Verification items for the finished model (mm, model axes). Face numbers are marked on the shaded views. Give positions to 0.01 mm unless a question says otherwise; leave off trailing zeros. Order: outer loops, then holes, each group sorted by start corner. A loop starts at its lowest first (then second) coordinate and runs counter-clockwise, first axis right, second up. Notation, with made-up numbers: M 16.25,59.25 L 70.25,59.25 A18 ccw 70.25,85.25 Z; hole C 3,-32 d3. An arc over 180 degrees is marked long. Answer as a JSON object with one key per item and string values.
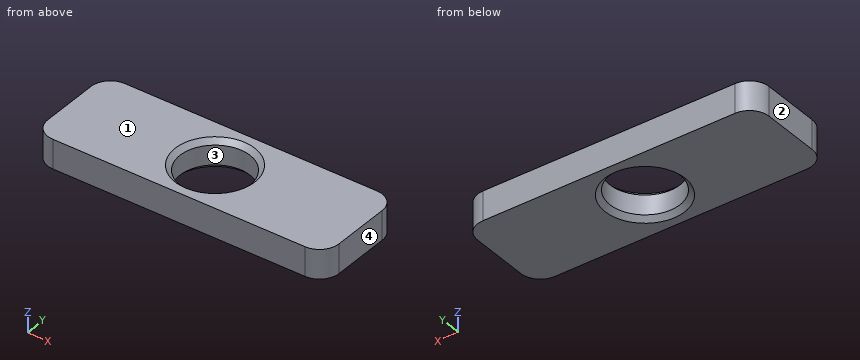
```python
from build123d import *

# Parameters (mm, degrees)
F0_W     = 300
F0_H     = 100
F0_R     = 36.023604
F1_DEPTH = 30
F2_R     = 20
F3_SIZE  = 5


with BuildPart() as f1:
    # F0 (on Top) → F1 (new body)
    with BuildSketch(Plane.XY):
        Rectangle(F0_W, F0_H)
        Circle(F0_R, mode=Mode.SUBTRACT)
    extrude(amount=F1_DEPTH)

    # F2
    f2_edges = [f1.edges().sort_by_distance(p)[0] for p in [
        (150, -50, 15),
        (150, 50, 15),
        (-150, -50, 15),
        (-150, 50, 15),
    ]]
    fillet(f2_edges, radius=F2_R)

    # F3
    f3_edges = [f1.edges().sort_by_distance(p)[0] for p in [
        (-36.023604, 0, 30),
        (-36.023604, 0, 0),
    ]]
    chamfer(f3_edges, length=F3_SIZE)


solid = f1.part
```
Q1. Release check for a two-part mould opening along X. For the marked faces 1, 2, 3 and 4 record: +X half, -X half, draft (parallel to the pull), parting line (faces both ways), or undercut.
Resolved:
{"face 1": "draft", "face 2": "-X half", "face 3": "undercut", "face 4": "+X half"}
Q2. Section check A-A on x = 0. Record the cut outline in (y, z), then the cut area to 3 significant figures.
Resolved:
{"outline": "M -50,0 L -41.02,0 L -36.02,5 L -36.02,25 L -41.02,30 L -50,30 Z; M 36.02,5 L 41.02,0 L 50,0 L 50,30 L 41.02,30 L 36.02,25 Z", "area": "789 mm²"}
Q3. Section check B-B on y = 0. Record the cut outline in (x, z).
Resolved:
{"outline": "M -150,0 L -41.02,0 L -36.02,5 L -36.02,25 L -41.02,30 L -150,30 Z; M 36.02,5 L 41.02,0 L 150,0 L 150,30 L 41.02,30 L 36.02,25 Z"}
Q4. Section check C-C on z = 10.5. Record the cut outline in (x, y).
Resolved:
{"outline": "M -150,-30 A20 ccw -130,-50 L 130,-50 A20 ccw 150,-30 L 150,30 A20 ccw 130,50 L -130,50 A20 ccw -150,30 Z; hole C 0,0 d72.05"}
Q5. Material ranges on L1, parallel to Y at x = 0, z = 12; L2, parallel to Y at x = -20, z = 22.5; L3, parallel to X at y = 1.5, z = 17, recorded low to high.
Resolved:
{"L1": "y = -50 to -36.02, 36.02 to 50", "L2": "y = -50 to -29.96, 29.96 to 50", "L3": "x = -150 to -35.99, 35.99 to 150"}
